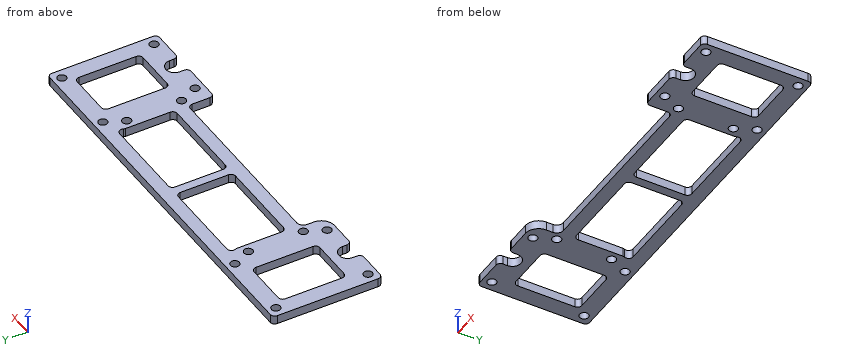
from build123d import *

# Parameters (mm, degrees)
SKETCH_1_W           = 176
SKETCH_1_H           = 50
EXTRUDE_1_DEPTH      = 2
SKETCH_2_R           = 2.025
CUT_EXTRUDE_1_DEPTH  = 22
CUT_EXTRUDE_2_DEPTH  = 17
FILLET_1_R           = 2
SKETCH_4_R           = 2.025
CUT_EXTRUDE_3_DEPTH  = 5
CUT_EXTRUDE_5_DEPTH  = 15.5
SKETCH_8_W           = 22.857142857
SKETCH_8_H           = 30
CUT_EXTRUDE_6_DEPTH  = 15.5
FILLET_2_R           = 2
SKETCH_22_W          = 54
SKETCH_22_H          = 23
CUT_EXTRUDE_14_DEPTH = 10
EXTRUDE_8_DEPTH      = 4
CHAMFER_1_SIZE       = 10
CHAMFER_2_SIZE       = 10
FILLET_9_R           = 2
SKETCH_24_W          = 87
SKETCH_24_H          = 30
CUT_EXTRUDE_15_DEPTH = 10
SKETCH_25_W          = 4
SKETCH_25_H          = 12
EXTRUDE_9_DEPTH      = 4
FILLET_10_R          = 2
CUT_EXTRUDE_16_DEPTH = 10


with BuildPart() as part:
    # 草图1 → 凸台-拉伸1 (new, symmetric)
    with BuildSketch(Plane.XY):
        Rectangle(SKETCH_1_W, SKETCH_1_H)
    extrude(amount=EXTRUDE_1_DEPTH, both=True)

    # 草图2 → 切除-拉伸1 (cut, symmetric)
    with BuildSketch(Plane(origin=(0, 0, -2), x_dir=(-1, 0, 0), z_dir=(0, 0, -1))):
        with Locations((51.5, 21)):
            Circle(SKETCH_2_R)
        with Locations((51.5, -21)):
            Circle(SKETCH_2_R)
        with Locations((83.5, 21)):
            Circle(SKETCH_2_R)
        with Locations((83.5, -21)):
            Circle(SKETCH_2_R)
    cut_extrude_1 = extrude(amount=CUT_EXTRUDE_1_DEPTH, both=True, mode=Mode.SUBTRACT)

    # 镜向1: 切除-拉伸1 across plane
    add(cut_extrude_1.mirror(Plane(origin=(0, 0, 0), x_dir=(0, 0, 1), z_dir=(1, 0, 0))), mode=Mode.SUBTRACT)

    # 草图3 → 切除-拉伸2 (cut, symmetric)
    with BuildSketch(Plane(origin=(0, 0, -2), x_dir=(-1, 0, 0), z_dir=(0, 0, -1))):
        with BuildLine():
            Line((63.5, -21), (63.5, -25))
            Line((63.5, -25), (71.5, -25))
            Line((71.5, -25), (71.5, -21))
            ThreePointArc((71.5, -21), (67.5, -17), (63.5, -21))
        make_face()
    cut_extrude_2 = extrude(amount=CUT_EXTRUDE_2_DEPTH, both=True, mode=Mode.SUBTRACT)

    # 镜向2: 切除-拉伸2 across plane
    add(cut_extrude_2.mirror(Plane(origin=(0, 0, 0), x_dir=(0, 0, 1), z_dir=(1, 0, 0))), mode=Mode.SUBTRACT)

    # 圆角1
    fillet_1_edges = [part.edges().sort_by_distance(p)[0] for p in [
        (-71.5, -25, 0),
        (-63.5, -25, 0),
        (88, -25, 0),
        (-88, -25, 0),
        (-88, 25, 0),
        (88, 25, 0),
        (63.5, -25, 0),
        (71.5, -25, 0),
    ]]
    fillet(fillet_1_edges, radius=FILLET_1_R)

    # 草图4 → 切除-拉伸3 (cut, symmetric)
    with BuildSketch(Plane(origin=(0, 0, -2), x_dir=(-1, 0, 0), z_dir=(0, 0, -1))):
        with Locations((47.5, -12.5)):
            Circle(SKETCH_4_R)
        with Locations((47.5, 12.5)):
            Circle(SKETCH_4_R)
        with Locations((-47.5, 12.5)):
            Circle(SKETCH_4_R)
        with Locations((-47.5, -12.5)):
            Circle(SKETCH_4_R)
    extrude(amount=CUT_EXTRUDE_3_DEPTH, both=True, mode=Mode.SUBTRACT)

    # 草图7 → 切除-拉伸5 (cut, symmetric)
    with BuildSketch(Plane.XY.offset(2)):
        Polygon((-2, 19), (-45.032854639, 19), (-43.5, 15.742683893), (-43.5, -15.742683893), (-45.032854639, -19), (-2, -19), align=None)
        Polygon((45.032854639, 19), (2, 19), (2, -19), (45.032854639, -19), (43.5, -15.742683893), (43.5, 15.742683893), align=None)
    extrude(amount=CUT_EXTRUDE_5_DEPTH, both=True, mode=Mode.SUBTRACT)

    # 草图8 → 切除-拉伸6 (cut, symmetric)
    with BuildSketch(Plane.XY.offset(2)):
        with Locations((-69.023809524, 2)):
            Rectangle(SKETCH_8_W, SKETCH_8_H)
        with Locations((69.023809524, 2)):
            Rectangle(SKETCH_8_W, SKETCH_8_H)
    extrude(amount=CUT_EXTRUDE_6_DEPTH, both=True, mode=Mode.SUBTRACT)

    # 圆角2
    fillet_2_edges = [part.edges().sort_by_distance(p)[0] for p in [
        (-2, 19, 0),
        (-2, -19, 0),
        (-45.032854639, -19, 0),
        (-43.5, -15.742683893, 0),
        (-43.5, 15.742683893, 0),
        (-45.032854639, 19, 0),
        (2, 19, 0),
        (45.032854639, 19, 0),
        (43.5, 15.742683893, 0),
        (43.5, -15.742683893, 0),
        (45.032854639, -19, 0),
        (2, -19, 0),
        (-80.452380952, -13, 0),
        (-80.452380952, 17, 0),
        (-57.595238095, 17, 0),
        (-57.595238095, -13, 0),
        (80.452380952, 17, 0),
        (80.452380952, -13, 0),
        (57.595238095, -13, 0),
        (57.595238095, 17, 0),
    ]]
    fillet(fillet_2_edges, radius=FILLET_2_R)

    # 草图22 → 切除-拉伸14 (cut)
    with BuildSketch(Plane(origin=(0, 0, -2), x_dir=(-1, 0, 0), z_dir=(0, 0, -1))):
        with Locations((0, -13.5)):
            Rectangle(SKETCH_22_W, SKETCH_22_H)
    extrude(amount=-CUT_EXTRUDE_14_DEPTH, mode=Mode.SUBTRACT)

    # 草图23 → 凸台-拉伸8 (add)
    with BuildSketch(Plane(origin=(0, 0, -2), x_dir=(-1, 0, 0), z_dir=(0, 0, -1))):
        Polygon((-31, -25), (-27, -25), (-27, -2), (27, -2), (27, -25), (31, -25), (31, 2), (-31, 2), align=None)
    extrude(amount=-EXTRUDE_8_DEPTH)

    # 倒角1
    chamfer_1_edges = [part.edges().sort_by_distance(p)[0] for p in [
        (27, -2, 0),
        (-27, -2, 0),
    ]]
    chamfer(chamfer_1_edges, length=CHAMFER_1_SIZE)

    # 倒角2
    chamfer_2_edges = [part.edges().sort_by_distance(p)[0] for p in [
        (31, 2, 0),
        (-31, 2, 0),
    ]]
    chamfer(chamfer_2_edges, length=CHAMFER_2_SIZE)

    # 圆角9
    fillet_9_edges = [part.edges().sort_by_distance(p)[0] for p in [
        (-27, -25, 0),
        (27, -25, 0),
        (-31, -19, 0),
        (-2, 2, 0),
        (31, -19, 0),
        (2, 2, 0),
        (21, 2, 0),
        (31, -8, 0),
        (-31, -8, 0),
        (-21, 2, 0),
    ]]
    fillet(fillet_9_edges, radius=FILLET_9_R)

    # 草图24 → 切除-拉伸15 (cut)
    with BuildSketch(Plane.XY.offset(2)):
        with Locations((0, -10)):
            Rectangle(SKETCH_24_W, SKETCH_24_H)
    extrude(amount=-CUT_EXTRUDE_15_DEPTH, mode=Mode.SUBTRACT)

    # 草图25 → 凸台-拉伸9 (add)
    with BuildSketch(Plane.XY.offset(2)):
        Polygon((2, -7), (-2, -7), (-43.5, -7), (-43.5, -13), (43.5, -13), (43.5, -7), align=None)
        with Locations((0, -1)):
            Rectangle(SKETCH_25_W, SKETCH_25_H)
        with BuildLine():
            Line((-43.5, -18.174640335), (-43.5, -15.295610336))
            ThreePointArc((-43.5, -15.295610336), (-43.548170754, -15.731915957), (-43.690362596, -16.147204408))
            Line((-43.690362596, -16.147204408), (-43.690928016, -16.148405927))
            ThreePointArc((-43.690928016, -16.148405927), (-43.872470388, -17.187624889), (-43.5, -18.174640335))
        make_face()
        with BuildLine():
            ThreePointArc((43.690362596, -16.147204408), (43.548170754, -15.731915957), (43.5, -15.295610336))
            Line((43.5, -15.295610336), (43.5, -18.174640335))
            ThreePointArc((43.5, -18.174640335), (43.872470388, -17.187624889), (43.690928016, -16.148405927))
            Line((43.690928016, -16.148405927), (43.690362596, -16.147204408))
        make_face()
    extrude(amount=-EXTRUDE_9_DEPTH)

    # 圆角10
    fillet_10_edges = [part.edges().sort_by_distance(p)[0] for p in [
        (-43.5, -25, 0),
        (43.5, -25, 0),
        (43.5, -7, 0),
        (43.5, -13, 0),
        (-43.5, -13, 0),
        (-43.5, -7, 0),
        (-2, -7, 0),
        (2, -7, 0),
    ]]
    fillet(fillet_10_edges, radius=FILLET_10_R)

    # 草图26 → 切除-拉伸16 (cut)
    with BuildSketch(Plane(origin=(0, 0, -2), x_dir=(-1, 0, 0), z_dir=(0, 0, -1))):
        with BuildLine():
            Line((44.5, -19), (44.5, -16))
            ThreePointArc((44.5, -16), (43.621320344, -13.878679656), (41.5, -13))
            ThreePointArc((41.5, -13), (42.914213562, -13.585786438), (43.5, -15))
            Line((43.5, -15), (43.5, -23))
            ThreePointArc((43.5, -23), (44.085786438, -24.414213562), (45.5, -25))
            Line((45.5, -25), (50.5, -25))
            ThreePointArc((50.5, -25), (46.257359313, -23.242640687), (44.5, -19))
        make_face()
    extrude(amount=-CUT_EXTRUDE_16_DEPTH, mode=Mode.SUBTRACT)


solid = part.part
Geometry: final body of the model. Coordinates: model frame, mm. Give positions to 0.01 mm unless a question says otherwise; leave off trailing zeros. Loops run counter-clockwise (first coordinate to the right, second up) from the corner with the lowest first, then second, coordinate; pieces in that order, holes last. Notation, with made-up numbers: (-9, 43) - (4, 43) arc R19 ccw to (4, 56) - close; hole circle Ø9 at (3.5, -4). An arc over 180 degrees is marked (long way). Answer as CSV lines item,"result". Start each with the question number.
1. Pin query (flat end, axial travel): P1, Ø1.5, axis at x = -41.5, z = -0.5, coming from the -Y side. Return the tip coordinate at first contact, or that it passes through.
2. Section D-D, the plane z = -1.4. Give the number of separate pieces and of enclosed holes in the cut face, plus the area to 3 significant figures.
3. Section C-C, the plane y = 0. Return loops of the section in (x, z), plus the area to 3 significant figures.
4. Ray query, L1, parallel to X at y = 5, z = 0.8; L2, parallel to Y at x = -83.5, z = 0 (3 decimals); L3, parallel to X at y = -10, z = 0.5. Return the intervals inside material, ascending.
5. Section A-A, the plane x = -35. Return loops of the section in (y, z).
6. Section B-B, the plane x = 51.5. Return loops of the section in (y, z) (3 decimals), plus the area to 3 significant figures.
Answers:
1,P1,"stops at y = -13.1"
2,separate pieces,"1"
2,enclosed holes,"16"
2,area,"3,940 mm2"
3,outline,"(-88, -2) - (-80.45, -2) - (-80.45, 2) - (-88, 2) - close; (-57.6, -2) - (-43.5, -2) - (-43.5, 2) - (-57.6, 2) - close; (-2, -2) - (2, -2) - (2, 2) - (-2, 2) - close; (43.5, -2) - (57.6, -2) - (57.6, 2) - (43.5, 2) - close; (80.45, -2) - (88, -2) - (88, 2) - (80.45, 2) - close"
3,area,"189 mm2"
4,L1,"x = -88 to -80.45, -57.6 to -43.5, -2 to 2, 43.5 to 57.6, 80.45 to 88"
4,L2,"y = -25 to -23.025, -18.975 to 18.975, 23.025 to 25"
4,L3,"x = -88 to -80.45, -57.6 to 57.6, 80.45 to 88"
5,outline,"(-13, -2) - (-7, -2) - (-7, 2) - (-13, 2) - close; (19, -2) - (25, -2) - (25, 2) - (19, 2) - close"
6,outline,"(-25, -2) - (-23.025, -2) - (-23.025, 2) - (-25, 2) - close; (-18.975, -2) - (18.975, -2) - (18.975, 2) - (-18.975, 2) - close; (23.025, -2) - (25, -2) - (25, 2) - (23.025, 2) - close"
6,area,"168 mm2"
